For this review, take the finished solid that the model builds, in its own axes (mm). A direction names the side the tool comes from. Give positions to 0.01 mm unless a question says otherwise; leave off trailing zeros. Loops run counter-clockwise (first coordinate to the right, second up) from the corner with the lowest first, then second, coordinate; pieces in that order, holes last.
Autodesk Inventor part; units mm, degrees
ref_plane "YZ Plane" through (0, 0, 0) normal (1, 0, 0) x (0, 1, 0)
ref_plane "XZ Plane" through (0, 0, 0) normal (0, 1, 0) x (-1, 0, 0)
ref_plane "XY Plane" through (0, 0, 0) normal (0, 0, 1) x (1, 0, 0)
sketch "Sketch1" plane through (0, 0, 0) normal (0, 1, 0) x (-1, 0, 0)
  line L0 (121, 0) -> (-97, 0) construction
  circle A0 centre (29, -10) radius 1.6
  circle A1 centre (69, -10) radius 1.6
  circle A2 centre (9, -60) radius 1.6
  circle A3 centre (-11, -60) radius 1.6
  line L1 (79, 0) -> (79, -20)
  line L2 (79, -20) -> (39, -20)
  line L3 (9, -71.9615) -> (-11, -71.9615)
  circle A4 centre (-31, -40) radius 1.6
  line L4 (-11, -71.9615) -> (-15.0192, -65)
  line L5 (-11, -71.9615) -> (19, -71.9615) construction
  circle A5 centre (-71, -40) radius 1.6
  line L6 (-49, -45.9808) -> (-81, -45.9808)
  line L7 (-81, -45.9808) -> (-81, -29.9998)
  line L8 (-81, -29.9998) -> (-11, -29.9998)
  line L9 (-11, -29.9998) -> (-1, -12.6793)
  line L10 (-1, -12.6793) -> (-1, 0)
  circle A6 centre (29, 10) radius 1.6
  circle A7 centre (69, 10) radius 1.6
  circle A8 centre (9, 60) radius 1.6
  circle A9 centre (-11, 60) radius 1.6
  line L11 (79, 0) -> (79, 20)
  line L12 (79, 20) -> (39, 20)
  line L13 (9, 71.9615) -> (-11, 71.9615)
  circle A10 centre (-31, 40) radius 1.6
  line L14 (-11, 71.9615) -> (-15.0192, 65)
  line L15 (-11, 71.9615) -> (19, 71.9615) construction
  circle A11 centre (-71, 40) radius 1.6
  line L16 (-49, 45.9808) -> (-81, 45.9808)
  line L17 (-81, 45.9808) -> (-81, 29.9998)
  line L18 (-81, 29.9998) -> (-11, 29.9998)
  line L19 (-11, 29.9998) -> (-1, 12.6793)
  line L20 (-1, 12.6793) -> (-1, 0)
  line L21 (-81, -45.9808) -> (-74, -45.9808)
  line L22 (-74, -45.9808) -> (-74, -29.9998)
  line L23 (-74, 29.9998) -> (-74, 45.9808)
  circle A12 centre (30.6, 40) radius 1.6
  arc A13 (33.0505, 30.3049) -> (23.429, 46.9697) centre (30.6, 40) ccw
  circle A14 centre (30.6, -40) radius 1.6
  arc A15 (23.429, -46.9697) -> (33.0505, -30.3049) centre (30.6, -40) ccw
  line L24 (39, 20) -> (33.0505, 30.3049)
  line L25 (23.429, 46.9697) -> (9, 71.9615)
  line L26 (39, -20) -> (33.0505, -30.3049)
  line L27 (23.429, -46.9697) -> (9, -71.9615)
  circle A16 centre (-36, 60) radius 1.6
  line L28 (-11, 60) -> (-11, 61.6)
  line L29 (-15.0192, 65) -> (-37.6, 65)
  line L30 (-37.6, 65) -> (-49, 45.9808)
  circle A17 centre (-36, -60) radius 1.6
  line L31 (-15.0192, -65) -> (-37.6, -65)
  line L32 (-37.6, -65) -> (-49, -45.9808)
  point P0 (0, 0)
  point P1 (-26, -45.9808)
  point P2 (-26, 45.9808)
  dimension "d0" = 3.2
  dimension "d3" = 3.2
  dimension "d5" = 3.2
  dimension "d6" = 50
  dimension "d15" = 20
  dimension "d16" = 40
  dimension "d18" = 20
  dimension "d25" = 3.2
  dimension "d27" = 40
  dimension "d28" = 120
  dimension "d29" = 3.2
  dimension "d30" = 40
  dimension "d31" = 55
  dimension "d32" = 15.981
  dimension "d33" = 120
  dimension "d36" = 3.2
  dimension "d37" = 30
  dimension "d38" = 20
  dimension "d39" = 3.2
  dimension "d40" = 25
extrude "Extrusion1" add sketch "Sketch1" along normal blind 4
sketch "Sketch2" plane through (0, 4, 0) normal (0, 1, 0) x (1, 0, 0)
  point P0 (0, 0)
extrude "Extrusion2" cut sketch "Sketch1" along normal blind 4 contours L6 L7 L8 L22 | L23 L18 L17 L16
fillet "Fillet1" radius 7 26 edges at (49, 2, 45.9808) (37.6, 2, 65) (74, 2, 45.9808) (74, 2, 29.9998) (1, 2, 12.6793) (1, 2, -12.6793) (11, 2, -29.9998) (11, 2, 29.9998) (74, 2, -29.9998) (49, 2, -45.9808) (74, 2, -45.9808) (37.6, 2, -65) (15.0192, 2, -65) (11, 2, -71.9615) (-9, 2, -71.9615) (-23.429, 2, -46.9697) (-33.0505, 2, -30.3049) (-39, 2, -20) (-79, 2, -20) (-79, 2, 20) (-33.0505, 2, 30.3049) (-39, 2, 20) (-23.429, 2, 46.9697) (-9, 2, 71.9615) (11, 2, 71.9615) (15.0192, 2, 65)
properties part number "Fix Konektor Casis_3DPrint"
Item 1: Tool access review of faces 1 (the cylindrical face through (-8.41, 2.03, -71.05)), 2 (the flat face through (-1, 4, 1)), 3 (the flat face through (1, 2, 0)), 4 (the cylindrical face through (-39.5, 2.03, 20.96)), 5 (the flat face through (26, 2, -65)): name each direction out of +Z, -Z, +X, -X, +Y, -Y from which nothing blocks a thin tool from reaching the whole face with its end or side.
Answer:
face 1: -Z, -X, +Y, -Y
face 2: +Z, -Z, +X, -X, +Y
face 3: +X, +Y, -Y
face 4: -X, +Y, -Y
face 5: -Z, +X, +Y, -Y
Item 2: Take a section at A-A on x = 50.5. Give the boundary of the cut face in (y, z), and give its area (3 significant figures).
Answer:
outline: (0, -46.43) - (4, -46.43) - (4, -30) - (0, -30) - close; (0, 30) - (4, 30) - (4, 46.43) - (0, 46.43) - close
area: 131 mm2
Item 3: For L1, parallel to Z at x = -9, y = 1.15; L2, parallel to Z at x = 11, y = 1.65; L3, parallel to Z at x = 36.5, y = 1.4, list the stretches that pass through material, from the lowest coordinate up.
Answer:
L1: z = -70.68 to -61.6, -58.4 to 58.4, 61.6 to 70.68
L2: z = -70.68 to -61.6, -58.4 to -28.72, 28.72 to 58.4, 61.6 to 70.68
L3: z = -64.39 to -61.52, -58.48 to -30, 30 to 58.48, 61.52 to 64.39
Item 4: Clearance check with flat-ended pins moving along their axes: pin 1 Ø3 at (x, z) = (31, 40) entering from -Y; pin 2 Ø1.2 at (x, y) = (32.5, 2) entering from -Z; pin 3 Ø1 at (x, y) = (39, 0.5) entering from +Z; pin 4 Ø1.2 at (x, y) = (63, 2.5) entering from -Z. State where each tip first meets the part, or that it passes through.
Answer:
pin 1: passes through
pin 2: stops at z = -65
pin 3: stops at z = 63.03
pin 4: stops at z = -45.98
Item 5: Take a section at B-B on y = 0.75. State how many separate pieces and enclosed holes the cut face has, and give its area (3 significant figures).
Answer:
separate pieces: 1
enclosed holes: 16
area: 10,300 mm2
Item 6: The part is to be moulded in two halves that separate along X. For faces 6 (the flat face through (-79, 2, 0)), 7 (the cylindrical face through (11.208, 1.972, -61.586)), 8 (the cylindrical face through (71.9, 2, -32)), say which applies: released by +X, released by -X, zero draft, split by the parting line, or undercut.
Answer:
face 6: released by -X
face 7: undercut
face 8: released by +X
